CAD build for the part. Positions are in the model's coordinates, mm. Give positions to 0.01 mm unless a question says otherwise; leave off trailing zeros. Order: outer loops, then holes, each group sorted by start corner. A loop starts at its lowest first (then second) coordinate and runs counter-clockwise, first axis right, second up. Notation, with made-up numbers: M 59,5 L 65,5 A29 ccw 65,31 Z; hole C 32.5,31.25 d3. An arc over 180 degrees is marked long. Put each result on its own line as item: value. Start each with the question number.
1) Pin check, flat tips, straight feed: pin 1 (12 mm diameter, centred on x = 25.5, y = 37.5, fed in from -Z); pin 2 (6 mm diameter, centred on y = 25.5, z = 20, fed in from +X); pin 3 (10 mm diameter, centred on x = 15.5, z = 3, fed in from -Y); pin 4 (1.5 mm diameter, centred on x = 6.5, z = 4, fed in from -Y). Stop position of each tip, or through.
2) Cut at D-D (z = 34). Write the cut outline in (x, y), and give its area (3 significant figures).
3) Cut at C-C (y = 38.5). Write the cut outline in (x, z), and give its area (3 significant figures).
4) Drill centre lines: line 1 (Z direction, x = 5, y = 34); line 2 (Y direction, x = 22, z = -9); line 3 (Y direction, x = 17, z = 17). Where is each one in solid material? Low to high. Write a range as [from, to].
5) Two-plate mould, pull along X, no slides. Class faces 1 (the face through (29, 22, 14)), 2 (the face through (13, 21.743, 23)), 3 (the face through (-3, 22, 14)): released by +X, released by -X, zero draft, split by the parting line, or undercut.
6) Cut at A-A (y = 28). Write the cut outline in (x, z), and give its area (3 significant figures).
```python
from build123d import *

# Parameters (mm, degrees)
F0_W         = 3
F0_H         = 20
F1_DEPTH     = 10
F2_W         = 3
F2_H         = 20
F3_DEPTH     = 3
F4_DEPTH     = 10
F6_DEPTH     = 25
F7_DEPTH     = 29
F8_R         = 2.99999
F9_R         = 1
F10_DEPTH    = 100
F11_R        = 40
F12_W        = 32
F12_H        = 1
F13_DEPTH    = 0.5
F14_T1_DEPTH = 36.3301270189
F15_SIZE     = 0.2


# Not quite as in the source:
# - a fillet or chamfer that OpenCascade refuses, or shapes differently, is made with other operations: its cross-section is extruded or revolved along the edge and cut away or added
# - a fillet or chamfer is up to 0.001 mm smaller than in the source, because OpenCascade refuses the exact size


with BuildPart() as f1:
    # F0 (on Right) → F1 (new body)
    with BuildSketch(Plane.YZ):
        with Locations((42.2427766025, 31.6474299499)):
            Rectangle(F0_W, F0_H)
    extrude(amount=F1_DEPTH)

    # F2 (on face) → F3 (join)
    with BuildSketch(Plane(origin=(0, 0, 0), x_dir=(0, -1, 0), z_dir=(-1, 0, 0))):
        with Locations((-42.2427766025, 31.6474299499)):
            Rectangle(F2_W, F2_H)
        Polygon((-28.7427766025, 41.6474299499), (-40.7427766025, 41.6474299499), (-40.7427766025, 21.6474299499), (-43.7427766025, 21.6474299499), (-43.7427766025, -18.3525700501), (-28.7427766025, -18.3525700501), (-18.7427766025, 6.6474299499), (-18.7427766025, 31.6474299499), align=None)
    extrude(amount=F3_DEPTH)

    # F4 (cut): a face of the model
    f4_faces = [f1.faces().sort_by_distance(p)[0] for p in [
        (10, 42.2427766025, 31.6474299499),
    ]]
    extrude(f4_faces, amount=-F4_DEPTH, mode=Mode.SUBTRACT)

    # F5 (on face) → F6 (cut)
    with BuildSketch(Plane.YZ):
        Polygon((33.2049743711, -13.3525700501), (26.7427766025, -13.3525700501), (28.7427766025, -18.3525700501), (34.3136367478, -16.124225992), align=None)
        Polygon((41.2427766025, -13.3525700501), (33.2049743711, -13.3525700501), (34.3136367478, -16.124225992), align=None)
        Polygon((34.3136367478, -16.124225992), (28.7427766025, -18.3525700501), (43.7427766025, -18.3525700501), (43.7427766025, -13.3525700501), (41.2427766025, -13.3525700501), align=None)
        Polygon((40.7427766025, 21.6474299499), (43.7427766025, 21.6474299499), (43.7427766025, 41.6474299499), (40.7427766025, 41.6474299499), (40.7427766025, 38.6474299499), align=None)
        Polygon((32.3136367478, -11.124225992), (33.2049743711, -13.3525700501), (41.2427766025, -13.3525700501), (43.7427766025, -12.3525700501), (43.7427766025, 21.6474299499), (40.7427766025, 21.6474299499), (40.7427766025, 38.6474299499), (31.7427766025, 38.6474299499), (29.9854172896, 38.6474299499), (21.7427766025, 30.4047892628), (21.7427766025, 28.6474299499), (21.7427766025, 15.3029243713), (24.3136367478, 8.875774008), align=None)
        Polygon((43.7427766025, -12.3525700501), (41.2427766025, -13.3525700501), (43.7427766025, -13.3525700501), align=None)
        Polygon((32.3136367478, -11.124225992), (26.7427766025, -13.3525700501), (33.2049743711, -13.3525700501), align=None)
    extrude(amount=-F6_DEPTH, mode=Mode.SUBTRACT)

    # F7 (add): a face of the model
    f7_faces = [f1.faces().sort_by_distance(p)[0] for p in [
        (0, 34.7427766025, 41.0550618211),
    ]]
    extrude(f7_faces, amount=F7_DEPTH)

    # F8 (radius 3 in the source; OpenCascade refuses exactly that, so slightly less here)
    f8_edges = [f1.edges().sort_by_distance(p)[0] for p in [
        (13, 26.742777, -13.35257),
        (13, 32.313637, -11.124226),
    ]]
    fillet(f8_edges, radius=F8_R)

    # F9 (on face) → F10 (cut)
    with BuildSketch(Plane.YZ.offset(29)):
        with Locations((28.4140346461, -9.4529679484)):
            Circle(F9_R)
    extrude(amount=-F10_DEPTH, mode=Mode.SUBTRACT)

    # F11
    f11_edges = [f1.edges().sort_by_distance(p)[0] for p in [
        (13, 18.742777, 6.64743),
    ]]
    fillet(f11_edges, radius=F11_R)

    # F12 (on face) → F13 (join)
    with BuildSketch(Plane(origin=(0, -6.4523266737, 6.4523266737), x_dir=(1, 0, 0), z_dir=(0, -0.7071067812, 0.7071067812))):
        with Locations((13, 36.1312567586)):
            Rectangle(F12_W, F12_H)
    extrude(amount=F13_DEPTH)

    # F14: fillet of radius 1 on 1 edges, made by hand

    # F14_s2 → F14_t1 (cut)
    with BuildSketch(Plane.YZ.offset(-5.1650635095)):
        with BuildLine():
            ThreePointArc((18.7427766025, 31.6474299499), (18.7427766025, 32.1650680401), (19.0015956476, 32.6133557762))
            Line((19.0015956476, 32.6133557762), (18.3892232119, 32.0009833405))
            Line((18.3892232119, 32.0009833405), (18.7427766025, 31.6474299499))
        make_face()
    extrude(amount=F14_T1_DEPTH, mode=Mode.SUBTRACT)

    # F15
    f15_edges = [f1.edges().sort_by_distance(p)[0] for p in [
        (13, 40.742777, 38.64743),
    ]]
    chamfer(f15_edges, length=F15_SIZE)


solid = f1.part
```
Solution:
1. pin 1: z = 38.65
1. pin 2: through
1. pin 3: y = 19.25
1. pin 4: y = 19.91
2. outline: M -3,21.1 L 29,21.1 L 29,25.34 L -3,25.34 Z
2. area: 136 mm²
3. outline: M -3,38.65 L 29,38.65 L 29,41.65 L -3,41.65 Z
3. area: 96.0 mm²
4. line 1: [38.65, 41.65]
4. line 2: [25, 27.52], [29.31, 31.38]
4. line 3: [18.74, 21.74]
5. face 1: released by +X
5. face 2: zero draft
5. face 3: released by -X
6. outline: M -3,-12.42 L 29,-12.42 L 29,-10.36 L -3,-10.36 Z; M -3,-8.54 L 29,-8.54 L 29,-0.34 L -3,-0.34 Z; M -3,36.66 L 29,36.66 L 29,40.9 L -3,40.9 Z
6. area: 464 mm²
